For this review, take the finished solid that the model builds, in its own axes (mm). A direction names the side the tool comes from. Round coordinates to 2 decimals unless told otherwise and drop trailing zeros. Write each loop counter-clockwise with the first axis right and the second up, starting at its lowest first coordinate (ties: lowest second). Pieces come first, ordered by that corner, then holes. Notation, with made-up numbers: (61, -33.75) -> (85, -33.75) arc R18 ccw to (85, -24.75) -> close; hole circle Ø6 at (68, 42). An arc over 180 degrees is marked (long way). Write item = value, one per line. Start each with the question number.
```python
from build123d import *

# Parameters (mm, degrees)
SKETCH2_R           = 10.85
SKETCH2_W           = 80
SKETCH2_H           = 9
BOSS_EXTRUDE1_DEPTH = 30


with BuildPart() as part:
    # Sketch2 → Boss-Extrude1 (new body)
    # profile 1 of 3: a face of its own
    with BuildSketch(Plane.XY):
        with BuildLine():
            ThreePointArc((0, 8), (2.343145751, 2.343145751), (8, 0))
            Line((8, 0), (32, 0))
            ThreePointArc((32, 0), (37.656854249, 2.343145751), (40, 8))
            Line((40, 8), (40, 21))
            Line((40, 21), (40, 30))
            Line((40, 30), (8, 30))
            ThreePointArc((8, 30), (2.343145751, 27.656854249), (0, 22))
            Line((0, 22), (0, 8))
        make_face()
        with Locations((20, 15)):
            Circle(SKETCH2_R, mode=Mode.SUBTRACT)
    # profile 2 of 3: a face of its own
    with BuildSketch(Plane.XY):
        with Locations((80, 25.5)):
            Rectangle(SKETCH2_W, SKETCH2_H)
    # profile 3 of 3: a face of its own
    with BuildSketch(Plane.XY):
        with BuildLine():
            Line((120, 30), (120, 21))
            Line((120, 21), (120, 8))
            ThreePointArc((120, 8), (122.343145751, 2.343145751), (128, 0))
            Line((128, 0), (152, 0))
            ThreePointArc((152, 0), (157.656854249, 2.343145751), (160, 8))
            Line((160, 8), (160, 22))
            ThreePointArc((160, 22), (157.656854249, 27.656854249), (152, 30))
            Line((152, 30), (120, 30))
        make_face()
        with Locations((140, 15)):
            Circle(SKETCH2_R, mode=Mode.SUBTRACT)
    extrude(amount=BOSS_EXTRUDE1_DEPTH)


solid = part.part
```
1. Consider section A-A, the plane x = 140. Give the boundary of the cut face in (y, z).
2. Consider section B-B, the plane y = 15. Give the boundary of the cut face in (x, z), then the cut area to 3 significant figures.
3. Machinability: for faces 1 (the flat face through (40, 14, 15)), 2 (the cylindrical face through (157.594, 2.281, 14.79)), which of the approach directions +Z, -Z, +X, -X, +Y, -Y give a long, thin tool a straight path to every point of the face, cutting with its end or side? Answer none if there is none.
4. Consider section D-D, the plane y = 24. Give the boundary of the cut face in (x, z), then the cut area to 3 significant figures.
5. Wall thickness on L1, parallel to Y at x = 140, z = 17; L2, parallel to X at y = 18, z = 20.25; L3, parallel to X at y = 14, z = 11.75: over which ranges is each line inside the solid? List them lowest first. Write a range as from..to.
6. Clearance check with flat-ended pins moving along their axes: pin 1 Ø4 at (y, z) = (27, 25) entering from -X; pin 2 Ø9 at (x, z) = (68.5, 9.5) entering from -Y. State where each tip first meets the part, or that it passes through.
7. Draft analysis for pull direction Y (two halves, no side actions). For faces 3 (the cylindrical face through (150.35, 18.26, 14.79)), 4 (the flat face through (79, 22, 0)), 5 (the cylindrical face through (2.281, 2.406, 14.79)), state which applies: +Y half, -Y half, draft (parallel to the pull), parting line (faces both ways), or undercut.
8. Consider section C-C, the plane z = 3. Give the boundary of the cut face in (x, y).
Outcome:
q1.outline = (0, 0) -> (4.15, 0) -> (4.15, 30) -> (0, 30) -> close; (25.85, 0) -> (30, 0) -> (30, 30) -> (25.85, 30) -> close
q2.outline = (0, 0) -> (9.15, 0) -> (9.15, 30) -> (0, 30) -> close; (30.85, 0) -> (40, 0) -> (40, 30) -> (30.85, 30) -> close; (120, 0) -> (129.15, 0) -> (129.15, 30) -> (120, 30) -> close; (150.85, 0) -> (160, 0) -> (160, 30) -> (150.85, 30) -> close
q2.area = 1,100 mm2
q3.face_1 = +Z, -Z, -Y
q3.face_2 = +Z, -Z, +X, -Y
q4.outline = (0.25, 0) -> (13.94, 0) -> (13.94, 30) -> (0.25, 30) -> close; (26.06, 0) -> (133.94, 0) -> (133.94, 30) -> (26.06, 30) -> close; (146.06, 0) -> (159.75, 0) -> (159.75, 30) -> (146.06, 30) -> close
q4.area = 4,060 mm2
q5.L1 = 0..4.15, 25.85..30
q5.L2 = 0..9.57, 30.43..40, 120..129.57, 150.43..160
q5.L3 = 0..9.2, 30.8..40, 120..129.2, 150.8..160
q6.pin_1 = 0.58
q6.pin_2 = 21
q7.face_3 = undercut
q7.face_4 = draft
q7.face_5 = -Y half
q8.outline = (0, 8) arc R8 ccw to (8, 0) -> (32, 0) arc R8 ccw to (40, 8) -> (40, 21) -> (120, 21) -> (120, 8) arc R8 ccw to (128, 0) -> (152, 0) arc R8 ccw to (160, 8) -> (160, 22) arc R8 ccw to (152, 30) -> (8, 30) arc R8 ccw to (0, 22) -> close; hole circle Ø21.7 at (20, 15); hole circle Ø21.7 at (140, 15)
